Can you work these out from the model? Positions are in its coordinate system, mm. A direction names the side the tool comes from. Round coordinates to 2 decimals unless told otherwise and drop trailing zeros. Loops run counter-clockwise (first coordinate to the right, second up) from the corner with the lowest first, then second, coordinate; pieces in that order, holes last.
(1) If I drill on line 1 along X through (y, z) = (-5.5, 50); line 2 along Y through (x, z) = (-148, 5.5); line 3 along Y through (x, z) = (-144, 6), over which ranges is the centre line in solid material (lowest first)?
(2) Which directions (+Z, -Z, +X, -X, +Y, -Y) give clear straight access to the entire face, cutting with the end or side of a thin tool? Please do faces 1 (the face through (-135.612, 0, 40)), 2 (the face through (-113.644, -16.074, 39.514)).
(3) Thinking about a two-plate mould opening in X: for faces 3 (the face through (-189.04, 17.42, 39.51)), 4 (the face through (-157.3, -12.4, 39.5)), 5 (the face through (-154.053, -39.543, 39.514)), 6 (the face through (-123.325, -29.472, 39.514)), which applies, released by +X, released by -X, zero draft, split by the parting line, or undercut?
(4) I want a section at A-A on x = -145.5. Write out the boundary of the cut face in (y, z), plus the area to 3 significant figures.
(5) I want a section at B-B on x = -174. Write out the boundary of the cut face in (y, z), plus the area to 3 significant figures.
(6) Will these pins go through, and if not, where does the flat tip stop? pin 1 Ø1.5 at (x, z) = (-169.5, 14.5) entering from -Y; pin 2 Ø5 at (y, z) = (-4, 31.5) entering from +X; pin 3 Ø12 at (y, z) = (16.5, 58.5) entering from +X.
from build123d import *

# Parameters (mm, degrees)
SKETCH004_R           = 42.75
PAD005_DEPTH          = 80.15
SKETCH005_R           = 10.478477
POCKET004_DEPTH       = 370.285607
POLARPATTERN004_COUNT = 15
POCKET016_DEPTH       = 80.151


with BuildPart() as part:
    # Sketch004 → Pad005 (new body)
    with BuildSketch(Plane.XY):
        Circle(SKETCH004_R)
    extrude(amount=PAD005_DEPTH)

    # Sketch005 → Pocket004 (cut, through all)
    with BuildSketch(Plane.XY):
        with Locations((50.228477, 0)):
            Circle(SKETCH005_R)
    pocket004 = extrude(amount=POCKET004_DEPTH, mode=Mode.SUBTRACT)

    # PolarPattern004: Pocket004 ×15 about axis
    polarpattern004_axis = Axis((0, 0, 0), (0, 0, 1))
    for i in range(1, POLARPATTERN004_COUNT):
        add(pocket004.rotate(polarpattern004_axis, i * 360 / POLARPATTERN004_COUNT), mode=Mode.SUBTRACT)

    # Sketch031 → Pocket016 (cut, through all)
    with BuildSketch(Plane.XY):
        Polygon((14.3875, 8.306627), (0, 16.613254), (-14.3875, 8.306627), (-14.3875, -8.306627), (0, -16.613254), (14.3875, -8.306627), align=None)
    extrude(amount=POCKET016_DEPTH, mode=Mode.SUBTRACT)


with BuildPart() as part_1:
    # Body010 placement: moved
    add(part.part.moved(Location((-150, 0, 0))))


solid = part_1.part
Filled sheet:
1. line 1: x = -189.89 to -164.39, -135.61 to -108.69
1. line 2: y = -42.39 to -15.46, 15.46 to 42.39
1. line 3: y = -42.33 to -13.15, 13.15 to 42.33
2. face 1: +Z, -Z
2. face 2: +Z, -Z, +X
3. face 3: released by -X
3. face 4: undercut
3. face 5: undercut
3. face 6: released by +X
4. outline: (-42.51, 0) - (-14.02, 0) - (-14.02, 80.15) - (-42.51, 80.15) - close; (14.02, 0) - (42.51, 0) - (42.51, 80.15) - (14.02, 80.15) - close
4. area: 4,570 mm2
5. outline: (-33.08, 0) - (33.08, 0) - (33.08, 80.15) - (-33.08, 80.15) - close
5. area: 5,300 mm2
6. pin 1: stops at y = -35.17
6. pin 2: stops at x = -107.99
6. pin 3: stops at x = -108.56
